from build123d import *

# Parameters (mm, degrees)
SKETCH1_R           = 2
BOSS_EXTRUDE1_DEPTH = 4
BOSS_EXTRUDE3_START = -1
SKETCH3_R           = 2
SKETCH3_R_2         = 1
BOSS_EXTRUDE3_DEPTH = 2
FILLET1_R           = 1


with BuildPart() as part:
    # Sketch1 → Boss-Extrude1 (new body)
    with BuildSketch(Plane.XY):
        with BuildLine():
            Line((-63.221147144, 4.5), (-2.221147144, 4.5))
            ThreePointArc((-2.221147144, 4.5), (1.924633844, -3.295084972), (-6.856271198, -2.375))
            ThreePointArc((-6.856271198, -2.375), (-7.960294648, -1.012531407), (-9.637345631, -0.5))
            Line((-9.637345631, -0.5), (-55.804948657, -0.5))
            ThreePointArc((-55.804948657, -0.5), (-57.48199964, -1.012531407), (-58.586023089, -2.375))
            ThreePointArc((-58.586023089, -2.375), (-67.366928132, -3.295084972), (-63.221147144, 4.5))
        make_face()
        with Locations((-63.221147144, -0.5)):
            Circle(SKETCH1_R, mode=Mode.SUBTRACT)
        with Locations((-2.221147144, -0.5)):
            Circle(SKETCH1_R, mode=Mode.SUBTRACT)
    extrude(amount=BOSS_EXTRUDE1_DEPTH)

    # Sketch3 → Boss-Extrude3 (add)
    with BuildSketch(Plane.XY.offset(4).offset(BOSS_EXTRUDE3_START)):
        with Locations((-17.221147144, -0.5)):
            Circle(SKETCH3_R)
        with Locations((-17.221147144, -0.5)):
            Circle(SKETCH3_R_2, mode=Mode.SUBTRACT)
    extrude(amount=-BOSS_EXTRUDE3_DEPTH)

    # Fillet1
    fillet1_edges = [part.edges().sort_by_distance(p)[0] for p in [
        (-15.221147144, -0.5, 2),
        (-19.221147144, -0.5, 2),
    ]]
    fillet(fillet1_edges, radius=FILLET1_R)


solid = part.part
Read the model definition and answer for the solid it produces. Units are mm, in the model's axes. A direction names the side the tool comes from. Coordinates: 2 decimals unless noted, no trailing zeros. Loops run counter-clockwise (first coordinate to the right, second up) from the corner with the lowest first, then second, coordinate; pieces in that order, holes last. Notation, with made-up numbers: (-0.5, -38) -> (38.5, -38) arc R17 ccw to (38.5, -28) -> close; hole circle Ø9 at (76.25, 84). An arc over 180 degrees is marked (long way). Answer in a Markdown table with one row per item.
Item 1: For faces 1 (the cylindrical face through (-67.28, -3.42, 1.97)), 2 (the cylindrical face through (-7.94, -1.027, 1.972)), 3 (the flat face through (-32, 1, 4)), 4 (the flat face through (-17, -2, 1)), 5 (the flat face through (-17, -2, 3)), determine the directions among +Z, -Z, +X, -X, +Y, -Y from which every point of the face is accessible in a straight line to the end or side of a thin tool.
Returned:
| item | result |
|---|---|
| face 1 | +Z, -Z |
| face 2 | +Z, -Z, -Y |
| face 3 | +Z, +X, -X, +Y, -Y |
| face 4 | -Z, -Y |
| face 5 | +Z, -Y |
Item 2: A cutting plane is placed at A-A on z = 1.8. Determine the outline of the cut face in (x, y) (3 decimals), plus the area to 3 significant figures.
Returned:
| item | result |
|---|---|
| outline | (-63.221, 4.5) arc R5 ccw (long way) to (-58.586, -2.375) arc R3 cw to (-55.805, -0.5) -> (-20.05, -0.5) arc R1 cw to (-19.107, -1.167) arc R2 ccw to (-15.336, -1.167) arc R1 cw to (-14.393, -0.5) -> (-9.637, -0.5) arc R3 cw to (-6.856, -2.375) arc R5 ccw (long way) to (-2.221, 4.5) -> close; hole circle Ø4 at (-63.221, -0.5); hole (-18.221, -0.5) arc R1 ccw to (-16.221, -0.5) -> close; hole circle Ø4 at (-2.221, -0.5) |
| area | 405 mm^2 |
Item 3: Each of these flat-tipped pins is pushed along its axis until it touches: P1, Ø2, axis at x = -50, z = 1, coming from the -Y side; P2, Ø0.6, axis at x = -16, y = -1.5, coming from the +Z side. Where does it stop, or does it pass through?
Returned:
| item | result |
|---|---|
| P1 | stops at y = -0.5 |
| P2 | stops at z = 3 |
Item 4: A cutting plane is placed at D-D on y = 3. Determine the outline of the cut face in (x, z), plus the area to 3 significant figures.
Returned:
| item | result |
|---|---|
| outline | (-66.79, 0) -> (1.35, 0) -> (1.35, 4) -> (-66.79, 4) -> close |
| area | 273 mm^2 |
Item 5: For a pull along X with two mould halves and no side action, classify faces 6 (the flat face through (-32, -0.5, 2)), 7 (the flat face through (-33, 4.5, 2)) as released by +X, released by -X, zero draft, split by the parting line, or undercut.
Returned:
| item | result |
|---|---|
| face 6 | undercut |
| face 7 | zero draft |
Item 6: A cutting plane is placed at B-B on y = -3.5. Determine the outline of the cut face in (x, z), plus the area to 3 significant figures.
Returned:
| item | result |
|---|---|
| outline | (-67.22, 0) -> (-59.22, 0) -> (-59.22, 4) -> (-67.22, 4) -> close; (-6.22, 0) -> (1.78, 0) -> (1.78, 4) -> (-6.22, 4) -> close |
| area | 64.0 mm^2 |
Item 7: A cutting plane is placed at C-C on x = -48. Determine the outline of the cut face in (y, z).
Returned:
| item | result |
|---|---|
| outline | (-0.5, 0) -> (4.5, 0) -> (4.5, 4) -> (-0.5, 4) -> close |
Item 8: Straight lines are drawn through the part: line 1 along X through (y, z) = (1.25, 1.45); line 2 along Y through (x, z) = (-49, 2.4); line 3 along X through (y, z) = (0, 1.65). For each, find the intervals that lie inside material, in ascending order. Write a range as [from, to].
Returned:
| item | result |
|---|---|
| line 1 | x = [-67.9, -64.19], [-62.25, -3.19], [-1.25, 2.46] |
| line 2 | y = [-0.5, 4.5] |
| line 3 | x = [-68.2, -65.16], [-61.28, -4.16], [-0.28, 2.75] |
